Check sheet for the modelled part. Datum: model origin and axes. Units: mm. Round coordinates to 2 decimals unless told otherwise and drop trailing zeros. Write each loop counter-clockwise with the first axis right and the second up, starting at its lowest first coordinate (ties: lowest second). Pieces come first, ordered by that corner, then holes.
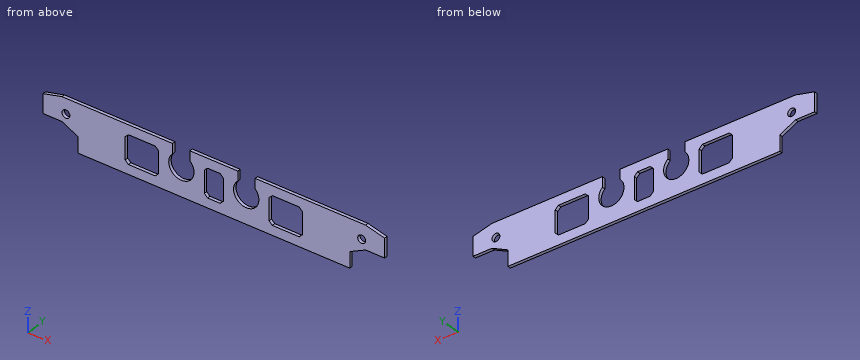
from build123d import *

# Parameters (mm, degrees)
CROQUIS1_W                = 86
CROQUIS1_H                = 15
SALIENTE_EXTRUIR1_DEPTH   = 1
CROQUIS2_W                = 6
CROQUIS2_H                = 9
CROQUIS2_W_2              = 10.5
CORTAR_EXTRUIR1_DEPTH     = 1
CHAFL_N1_SIZE             = 1
CORTAR_EXTRUIR2_DEPTH     = 1
CROQUIS4_R                = 1.25
SALIENTE_EXTRUIR2_DEPTH   = 1
SALIENTE_EXTRUIR2_2_DEPTH = 1


with BuildPart() as part:
    # Croquis1 → Saliente-Extruir1 (new body)
    with BuildSketch(Plane(origin=(0, 0, 0), x_dir=(1, 0, 0), z_dir=(0, 1, 0))):
        Rectangle(CROQUIS1_W, CROQUIS1_H)
    extrude(amount=SALIENTE_EXTRUIR1_DEPTH)

    # Croquis2 → Cortar-Extruir1 (cut)
    with BuildSketch(Plane(origin=(0, 1, 0), x_dir=(1, 0, 0), z_dir=(0, 1, 0))):
        Rectangle(CROQUIS2_W, CROQUIS2_H)
        with Locations((22.75, 0)):
            Rectangle(CROQUIS2_W_2, CROQUIS2_H)
        with Locations((-22.75, 0)):
            Rectangle(CROQUIS2_W_2, CROQUIS2_H)
    extrude(amount=-CORTAR_EXTRUIR1_DEPTH, mode=Mode.SUBTRACT)

    # Chafl_n1
    chafl_n1_edges = [part.edges().sort_by_distance(p)[0] for p in [
        (-17.5, 0.5, -4.5),
        (-17.5, 0.5, 4.5),
        (-28, 0.5, 4.5),
        (-28, 0.5, -4.5),
        (28, 0.5, -4.5),
        (28, 0.5, 4.5),
        (17.5, 0.5, 4.5),
        (17.5, 0.5, -4.5),
        (3, 0.5, -4.5),
        (3, 0.5, 4.5),
        (-3, 0.5, 4.5),
        (-3, 0.5, -4.5),
    ]]
    chamfer(chafl_n1_edges, length=CHAFL_N1_SIZE)

    # Croquis3 → Cortar-Extruir2 (cut)
    with BuildSketch(Plane(origin=(0, 1, 0), x_dir=(1, 0, 0), z_dir=(0, 1, 0))):
        with BuildLine():
            Line((-13.078515717, -7.5), (-7.578515717, -7.5))
            Line((-7.578515717, -7.5), (-7.578515717, -4.477107947))
            ThreePointArc((-7.578515717, -4.477107947), (-10.141843619, 2.498537507), (-13.078515717, -4.32833853))
            Line((-13.078515717, -4.32833853), (-13.078515717, -7.5))
        make_face()
        with BuildLine():
            Line((7.578515717, -7.5), (7.578515717, -4.477107947))
            ThreePointArc((7.578515717, -4.477107947), (10.141843619, 2.498537507), (13.078515717, -4.32833853))
            Line((13.078515717, -4.32833853), (13.078515717, -7.5))
            Line((13.078515717, -7.5), (7.578515717, -7.5))
        make_face()
    extrude(amount=-CORTAR_EXTRUIR2_DEPTH, mode=Mode.SUBTRACT)


with BuildPart() as body_2:
    # Croquis4 → Saliente-Extruir2 (new body)
    with BuildSketch(Plane(origin=(0, 1, 0), x_dir=(1, 0, 0), z_dir=(0, 1, 0))):
        Polygon((43, 2.5), (48, 0), (54, 0), (54, -6), (48, -7.5), (43, -7.5), align=None)
        with Locations(Location((46.75, -2.75, 0), (0, 0, 270))):
            Circle(CROQUIS4_R, mode=Mode.SUBTRACT)
    extrude(amount=-SALIENTE_EXTRUIR2_DEPTH)


with BuildPart() as body_3:
    # Croquis4 → Saliente-Extruir2 2 (new body)
    with BuildSketch(Plane(origin=(0, 1, 0), x_dir=(1, 0, 0), z_dir=(0, 1, 0))):
        Polygon((-43, 2.5), (-48, 0), (-54, 0), (-54, -6), (-48, -7.5), (-43, -7.5), align=None)
        with Locations(Location((-46.75, -2.75, 0), (0, 0, 90))):
            Circle(CROQUIS4_R, mode=Mode.SUBTRACT)
    extrude(amount=-SALIENTE_EXTRUIR2_2_DEPTH)


with BuildPart() as part_1:
    add(part.part)

    # Combinar1: union body 2, body 3
    add(body_2.part)
    add(body_3.part)


solid = part_1.part
1. Sectioned sample at A-A, the plane x = -24. Enter the section's corners in (y, z).
2. Sectioned sample at D-D, the plane x = -10.25. Enter the section's corners in (y, z).
3. Go/stop test with flat-tipped pins: pin 1 (0.5 mm diameter, centred on y = 0.5, z = -5.5, fed in from -X); pin 2 (1.5 mm diameter, centred on x = 9, z = -1, fed in from +Y); pin 3 (0.5 mm diameter, centred on y = 0.5, z = -6, fed in from +X); pin 4 (0.5 mm diameter, centred on y = 0.5, z = -1, fed in from +X). Record where each tip stops, or that it passes through.
4. Sectioned sample at B-B, the plane z = 2.5. Give the number of separate pieces and of enclosed holes in the cut face, plus the area to 3 significant figures.
5. Scan lines: line 1 along X through (y, z) = (0.6, -3); line 2 along Z through (x, y) = (19.5, 0.9); line 3 along X through (y, z) = (0.35, -0.25). Record each from-to range of solid material in increasing order.
Computed values:
1. outline: (0, -7.5) - (1, -7.5) - (1, -4.5) - (0, -4.5) - close; (0, 4.5) - (1, 4.5) - (1, 7.5) - (0, 7.5) - close
2. outline: (0, -7.5) - (1, -7.5) - (1, -2.5) - (0, -2.5) - close
3. pin 1: stops at x = -43
3. pin 2: passes through
3. pin 3: stops at x = 43
3. pin 4: stops at x = 46.5
4. separate pieces: 8
4. enclosed holes: 0
4. area: 60.6 mm2
5. line 1: x = -43 to -28, -17.5 to -3, 3 to 17.5, 28 to 43
5. line 2: z = -7.5 to -4.5, 4.5 to 7.5
5. line 3: x = -47.5 to -28, -17.5 to -13.85, -6.65 to -3, 3 to 6.65, 13.85 to 17.5, 28 to 47.5
